```python
from build123d import *

# Parameters (mm, degrees)
SKETCH2_R               = 2.8
SKETCH2_R_2             = 1.1
BOSS_EXTRUDE1_DEPTH     = 2.5
FILLET1_R               = 2.5
SKETCH4_R               = 17.25
SKETCH4_R_2             = 9.75
BOSS_EXTRUDE2_DEPTH     = 0.5
CUT_EXTRUDE1_DEPTH      = 37.267099556
CUT_EXTRUDE1_DEPTH_BACK = 37.267099556
SKETCH6_R               = 1.1


with BuildPart() as part:
    # Sketch1 → Revolve1 (revolve)
    with BuildSketch(Plane.XY, mode=Mode.PRIVATE) as revolve1_sk:
        Polygon((-2.5, 0), (0, 0), (0, 24.25), (-2.5, 24.25), (-2.5, 19), align=None)
    revolve(revolve1_sk.sketch.rotate(Axis((0, 0, 0), (-1, 0, 0)), 90), axis=Axis((0, 0, 0), (-1, 0, 0)))

    # Sketch2 → Boss-Extrude1 (add)
    # profile 1 of 2: a face of its own
    with BuildSketch(Plane(origin=(0, 0, 0), x_dir=(0, 0, -1), z_dir=(1, 0, 0))):
        with Locations((-24, 0)):
            Circle(SKETCH2_R)
        with Locations((-24, 0)):
            Circle(SKETCH2_R_2, mode=Mode.SUBTRACT)
    # profile 2 of 2: a face of its own
    with BuildSketch(Plane(origin=(0, 0, 0), x_dir=(0, 0, -1), z_dir=(1, 0, 0))):
        with Locations((24, 0)):
            Circle(SKETCH2_R)
        with Locations((24, 0)):
            Circle(SKETCH2_R_2, mode=Mode.SUBTRACT)
    extrude(amount=-BOSS_EXTRUDE1_DEPTH)

    # Fillet1
    fillet1_edges = [part.edges().sort_by_distance(p)[0] for p in [
        (-1.25, 2.798617784, 24.08796875),
        (-1.25, -2.798617784, 24.08796875),
        (-1.25, -2.798617784, -24.08796875),
        (-1.25, 2.798617784, -24.08796875),
    ]]
    fillet(fillet1_edges, radius=FILLET1_R)

    # Sketch4 → Boss-Extrude2 (add)
    with BuildSketch(Plane.ZY.offset(2.5)):
        Circle(SKETCH4_R)
        Circle(SKETCH4_R_2, mode=Mode.SUBTRACT)
    extrude(amount=BOSS_EXTRUDE2_DEPTH)

    # Sketch6 → Cut-Extrude1 (cut, two sides: drawn at the far end of the back side and taken through both)
    with BuildSketch(Plane(origin=(0, 0, 0), x_dir=(0, 0, -1), z_dir=(1, 0, 0)).offset(-CUT_EXTRUDE1_DEPTH_BACK)):
        with Locations((-24, 0)):
            Circle(SKETCH6_R)
        with Locations(Location((24, 0, 0), (0, 0, 180))):
            Circle(SKETCH6_R)
    extrude(amount=CUT_EXTRUDE1_DEPTH + CUT_EXTRUDE1_DEPTH_BACK, mode=Mode.SUBTRACT)


solid = part.part
```
Can you work these out from the model? Positions are in its coordinate system, mm. A direction names the side the tool comes from. Coordinates: 2 decimals unless noted, no trailing zeros. Order: outer loops, then holes, each group sorted by start corner. A loop starts at its lowest first (then second) coordinate and runs counter-clockwise, first axis right, second up. Notation, with made-up numbers: (36, -4) - (94, -4) arc R27 ccw to (94, 21) - close; hole circle Ø8 at (65, 7.25). An arc over 180 degrees is marked (long way). Answer in a Markdown table with one row per item.
1. Suppose I cut it at A-A (y = 0). Please give me the cut outline in (x, z).
Reply:
| item | result |
|---|---|
| outline | (-3, -17.25) - (-2.5, -17.25) - (-2.5, -22.9) - (0, -22.9) - (0, 22.9) - (-2.5, 22.9) - (-2.5, 17.25) - (-3, 17.25) - (-3, 9.75) - (-2.5, 9.75) - (-2.5, -9.75) - (-3, -9.75) - close; (-2.5, -26.8) - (0, -26.8) - (0, -25.1) - (-2.5, -25.1) - close; (-2.5, 25.1) - (0, 25.1) - (0, 26.8) - (-2.5, 26.8) - close |
2. Suppose I cut it at B-B (z = 12). Please give me the cut outline in (x, y), and give its area (3 significant figures).
Reply:
| item | result |
|---|---|
| outline | (-3, -12.39) - (-2.5, -12.39) - (-2.5, -21.07) - (0, -21.07) - (0, 21.07) - (-2.5, 21.07) - (-2.5, 12.39) - (-3, 12.39) - close |
| area | 118 mm^2 |
3. Suppose I cut it at D-D (y = 16). Please give me the cut outline in (x, z).
Reply:
| item | result |
|---|---|
| outline | (-3, -6.45) - (-2.5, -6.45) - (-2.5, -18.22) - (0, -18.22) - (0, 18.22) - (-2.5, 18.22) - (-2.5, 6.45) - (-3, 6.45) - close |
4. If I drill on line 1 along X through (y, z) = (6.5, 2); line 2 along Z through (x, y) = (-0.8, -3); line 3 along Z through (x, y) = (-0.7, 8), over which ranges is the centre line in solid material (lowest first)?
Reply:
| item | result |
|---|---|
| line 1 | x = -2.5 to 0 |
| line 2 | z = -24.55 to 24.55 |
| line 3 | z = -22.89 to 22.89 |
5. For faces 5 (the flat face through (-2.5, 0, 0)), 6 (the flat face through (-3, -7.4, 7.4)), which set-ups out of +Z, -Z, +X, -X, +Y, -Y let a thin tool reach every point of the face, with its end or its side?
Reply:
| item | result |
|---|---|
| face 5 | -X |
| face 6 | +Z, -Z, -X, +Y, -Y |
6. Suppose I cut it at C-C (x = -1). Give the number of separate pieces and of enclosed holes in the cut face, and give its area (3 significant figures).
Reply:
| item | result |
|---|---|
| separate pieces | 1 |
| enclosed holes | 2 |
| area | 1,860 mm^2 |
7. For pin 1 (1 mm diameter, centred on x = -1.5, y = 17.5, fed in from -Z); pin 2 (6 mm diameter, centred on y = -3, z = -4.5, fed in from -X); pin 3 (1 mm diameter, centred on x = -0.5, z = -18, fed in from +Y), each with a flat end and sliding along its axis, tell me the tip position at first contact or that it passes through.
Reply:
| item | result |
|---|---|
| pin 1 | stops at z = -17.29 |
| pin 2 | stops at x = -2.5 |
| pin 3 | stops at y = 16.79 |
8. If we mould it in two halves opening along Y, with no side actions, what happens to faces 1 (the cylindrical face through (-1.268, -24.245, -0.472)), 2 (the flat face through (-2.5, -14.3, 10.1)), 3 (the cylindrical face through (-1.2, 0, 25.1)), 4 (the cylindrical face through (-2.746, 9.667, -1.269))? For each: pulls with the +Y half, pulls with the -Y half, needs draft (parallel to the pull), parting line crosses it, or undercut.
Reply:
| item | result |
|---|---|
| face 1 | pulls with the -Y half |
| face 2 | needs draft |
| face 3 | undercut |
| face 4 | undercut |
